Read the model definition and answer for the solid it produces. Units are mm, in the model's axes. A direction names the side the tool comes from. Coordinates: 2 decimals unless noted, no trailing zeros. Order: outer loops, then holes, each group sorted by start corner. A loop starts at its lowest first (then second) coordinate and runs counter-clockwise, first axis right, second up.
```python
from build123d import *

# Parameters (mm, degrees)
SKETCH1_R           = 46
SKETCH1_R_2         = 43
BOSS_EXTRUDE1_DEPTH = 55
BOSS_EXTRUDE2_START = 3
BOSS_EXTRUDE2_DEPTH = 3
CUT_EXTRUDE1_DEPTH  = 58
BOSS_EXTRUDE3_START = -3
BOSS_EXTRUDE3_DEPTH = 3


with BuildPart() as part:
    # Sketch1 → Boss-Extrude1 (new body)
    with BuildSketch(Plane.XY):
        Circle(SKETCH1_R)
        Circle(SKETCH1_R_2, mode=Mode.SUBTRACT)
    extrude(amount=BOSS_EXTRUDE1_DEPTH)

    # Sketch2 → Boss-Extrude2 (add)
    with BuildSketch(Plane(origin=(0, 0, 0), x_dir=(-1, 0, 0), z_dir=(0, 0, -1)).offset(BOSS_EXTRUDE2_START)):
        with BuildLine():
            Line((-10, 17.320508076), (-23, 39.837168574))
            ThreePointArc((-23, 39.837168574), (23, 39.837168574), (46, 0))
            Line((46, 0), (20, 0))
            ThreePointArc((20, 0), (10, 17.320508076), (-10, 17.320508076))
        make_face()
    extrude(amount=-BOSS_EXTRUDE2_DEPTH)

    # Sketch3 → Cut-Extrude1 (cut)
    with BuildSketch(Plane(origin=(0, 0, -3), x_dir=(-1, 0, 0), z_dir=(0, 0, -1))):
        with BuildLine():
            Line((-23, 39.837168574), (-21.5, 37.239092363))
            ThreePointArc((-21.5, 37.239092363), (-21.5, -37.239092363), (43, 0))
            Line((43, 0), (46, 0))
            ThreePointArc((46, 0), (-23, -39.837168574), (-23, 39.837168574))
        make_face()
    extrude(amount=-CUT_EXTRUDE1_DEPTH, mode=Mode.SUBTRACT)

    # Sketch4 → Boss-Extrude3 (add)
    with BuildSketch(Plane.XY.offset(55).offset(BOSS_EXTRUDE3_START)):
        with BuildLine():
            Line((-37.239092363, 21.5), (-54.559600438, 31.5))
            Line((-54.559600438, 31.5), (-16.305599841, 60.853327056))
            Line((-16.305599841, 60.853327056), (-11.129218939, 41.53481053))
            ThreePointArc((-11.129218939, 41.53481053), (-26.176741447, 34.114193633), (-37.239092363, 21.5))
        make_face()
    extrude(amount=BOSS_EXTRUDE3_DEPTH)


solid = part.part
```
1) A cutting plane is placed at D-D, the plane x = -29. Determine the outline of the cut face in (y, z), and give its area (3 significant figures).
A:
outline: (0, -3) - (35.71, -3) - (35.71, 52) - (51.11, 52) - (51.11, 55) - (31.75, 55) - (31.75, 0) - (0, 0) - close
area: 371 mm2
2) A cutting plane is placed at A-A, the plane x = -44. Determine the outline of the cut face in (y, z).
A:
outline: (0, -3) - (13.42, -3) - (13.42, 55) - (0, 55) - close; (25.4, 52) - (39.6, 52) - (39.6, 55) - (25.4, 55) - close
3) A cutting plane is placed at C-C, the plane z = 28. Determine the outline of the cut face in (x, y).
A:
outline: (-46, 0) - (-43, 0) arc R43 cw to (21.5, 37.24) - (23, 39.84) arc R46 ccw to start
4) A cutting plane is placed at B-B, the plane y = 33. Determine the outline of the cut face in (x, z).
A:
outline: (-52.6, 52) - (-32.05, 52) - (-32.05, -3) - (19.05, -3) - (19.05, 0) - (-27.57, 0) - (-27.57, 55) - (-52.6, 55) - close
5) Which of the six approach directions +Z, -Z, +X, -X, +Y, -Y give full straight-line access (tool end or side, diameter ignored) to faces 1 (the cylindrical face through (-10.253, 17.172, -1.521)), 2 (the flat face through (-47.095, 27.19, 53.479)), 3 (the flat face through (-32, 41, 52)), 4 (the cylindrical face through (-20.95, 37.55, 27.12)), 5 (the flat face through (-12, 23, -3))?
A:
face 1: +Z, -Z, -Y
face 2: +Z, -Z, -X
face 3: -Z, -X, +Y
face 4: +Z, -Y
face 5: -Z, +X, -X, +Y, -Y
6) Flat-ended cylindrical pins translate along their axes: pin 1 Ø13 at (x, y) = (-24, 19) entering from +Z; pin 2 Ø8 at (y, z) = (29, 22.5) entering from -X; pin 3 Ø8 at (y, z) = (14.5, 24.5) entering from -X. Find the tip coordinate at first contact, or state that the pin passes through.
A:
pin 1: stops at z = 0
pin 2: stops at x = -38.61
pin 3: stops at x = -44.79
7) Straight lines are drawn through the part: line 1 (Z direction, x = -40, y = 8); line 2 (Y direction, x = -1, z = 11); line 3 (Z direction, x = -48, y = 28.5). For each, find the intervals that lie inside material, in ascending order.
A:
line 1: z = -3 to 0
line 2: y = 42.99 to 45.99
line 3: z = 52 to 55
